Can you work these out from the model? Positions are in its coordinate system, mm. A direction names the side the tool comes from. Coordinates: 2 decimals unless noted, no trailing zeros. Order: outer loops, then holes, each group sorted by start corner. A loop starts at its lowest first (then second) coordinate and runs counter-clockwise, first axis right, second up. Notation, with made-up numbers: (-5, 31) - (42, 31) arc R18 ccw to (42, 62) - close; hole circle Ø4 at (85, -39.5). An arc over 180 degrees is marked (long way). Use a Markdown table: item, result. Add a question column.
(1) I want a section at C-C (y = 3.75). List the corners of the cut face in (x, z) for me, and give its area (3 significant figures).
(2) I want a section at D-D (x = 0). List the corners of the cut face in (y, z) for me, and give its area (3 significant figures).
(3) I want a section at B-B (y = 19). List the corners of the cut face in (x, z) for me.
(4) For pin 1 Ø9 at (x, y) = (-18.5, 7) entering from -Z; pin 2 Ø5 at (y, z) = (18, 35) entering from +X; pin 3 Ø2 at (x, y) = (-27, 7.5) entering from -Z; pin 4 Ø6 at (x, y) = (8.5, 11) entering from +Z, each with a flat end and sliding along its axis, tell me the tip position at first contact or that it passes through.
(5) We'd pull the mould along X, two halves only. Please class faces 5 (the cylindrical face through (25.74, 6.26, 27.16)), 6 (the flat face through (-20.32, 18, 33)), 7 (the flat face through (-15, 22.86, 33)), 8 (the cylindrical face through (1.72, 6.26, -50.77)): pulls with the +X half, pulls with the -X half, needs draft (parallel to the pull), parting line crosses it, or undercut.
(6) If I drill on L1, parallel to X at y = 9.5, z = 0; L2, parallel to Y at x = 42.5, z = 2.5; L3, parallel to X at y = 6.5, z = 6, over which ranges is the centre line in solid material (lowest first)? Write a range as [from, to].
(7) On a 3-axis mill with a long thin cutter (end or side, diameter ignored), from which of +Z, -Z, +X, -X, +Y, -Y can I reach the whole of each face in a straight line? I mean faces 1 (the flat face through (-10.16, 11, 33)), 2 (the flat face through (-15, 0, -36)), 3 (the flat face through (20.32, 18, 33)), 4 (the flat face through (16, 11, 28.137)). Say none if no direction works.
(8) I want a section at A-A (z = 0). List the corners of the cut face in (x, y) for me, and give its area (3 significant figures).
```python
from build123d import *

# Parameters (mm, degrees)
SKETCH1_R           = 50.8
BOSS_EXTRUDE1_DEPTH = 12.7
CUT_EXTRUDE1_DEPTH  = 12.7
SKETCH3_W           = 10.16
SKETCH3_H           = 10.16
BOSS_EXTRUDE2_DEPTH = 10.16
FILLET1_R           = 10.16
FILLET2_R           = 10.16


with BuildPart() as part:
    # Sketch1 → Boss-Extrude1 (new body)
    with BuildSketch(Plane(origin=(0, 0, 0), x_dir=(1, 0, 0), z_dir=(0, 1, 0))):
        Circle(SKETCH1_R)
    extrude(amount=BOSS_EXTRUDE1_DEPTH)

    # Sketch2 → Cut-Extrude1 (cut)
    with BuildSketch(Plane(origin=(0, 12.7, 0), x_dir=(1, 0, 0), z_dir=(0, 1, 0))):
        with BuildLine():
            Line((-25.689206411, -28.136713987), (-10.16, -28.136713987))
            Line((-10.16, -28.136713987), (-10.16, -38.296713987))
            Line((-10.16, -38.296713987), (-33.376663971, -38.296713987))
            ThreePointArc((-33.376663971, -38.296713987), (0, -50.8), (33.376663971, -38.296713987))
            Line((33.376663971, -38.296713987), (10.16, -38.296713987))
            Line((10.16, -38.296713987), (10.16, -28.136713987))
            Line((10.16, -28.136713987), (25.689206411, -28.136713987))
            ThreePointArc((25.689206411, -28.136713987), (0, 38.1), (-25.689206411, -28.136713987))
        make_face()
    extrude(amount=-CUT_EXTRUDE1_DEPTH, mode=Mode.SUBTRACT)

    # Sketch3 → Boss-Extrude2 (add)
    with BuildSketch(Plane(origin=(-12.7, 12.7, 0), x_dir=(0, 0, -1), z_dir=(0, -1, 0))):
        with Locations((-33.216713987, -2.54)):
            Rectangle(SKETCH3_W, SKETCH3_H)
    boss_extrude2 = extrude(amount=-BOSS_EXTRUDE2_DEPTH)

    # Fillet1
    fillet1_edges = [part.edges().sort_by_distance(p)[0] for p in [
        (-25.689206411, 6.35, 28.136713987),
    ]]
    fillet(fillet1_edges, radius=FILLET1_R)

    # Mirror1: Boss-Extrude2 across plane
    add(boss_extrude2.mirror(Plane(origin=(0, 0, 0), x_dir=(0, 0, 1), z_dir=(1, 0, 0))))

    # Fillet2
    fillet2_edges = [part.edges().sort_by_distance(p)[0] for p in [
        (25.689206411, 6.35, 28.136713987),
    ]]
    fillet(fillet2_edges, radius=FILLET2_R)


solid = part.part
```
Answers follow:
| question | item | result |
|---|---|---|
| 1 | outline | (-33.38, 38.3) arc R50.8 ccw (long way) to (33.38, 38.3) - (10.16, 38.3) - (10.16, 28.14) - (21.39, 28.14) arc R10.16 cw to (29.17, 24.51) arc R38.1 cw (long way) to (-29.17, 24.51) arc R10.16 cw to (-21.39, 28.14) - (-10.16, 28.14) - (-10.16, 38.3) - close |
| 1 | area | 3,130 mm² |
| 2 | outline | (0, -50.8) - (12.7, -50.8) - (12.7, -38.1) - (0, -38.1) - close |
| 2 | area | 161 mm² |
| 3 | outline | (-20.32, 28.14) - (-10.16, 28.14) - (-10.16, 38.3) - (-20.32, 38.3) - close; (10.16, 28.14) - (20.32, 28.14) - (20.32, 38.3) - (10.16, 38.3) - close |
| 4 | pin 1 | stops at z = -48.83 |
| 4 | pin 2 | stops at x = 20.32 |
| 4 | pin 3 | stops at z = -43.64 |
| 4 | pin 4 | stops at z = 38.3 |
| 5 | face 5 | undercut |
| 5 | face 6 | pulls with the -X half |
| 5 | face 7 | needs draft |
| 5 | face 8 | parting line crosses it |
| 6 | L1 | x = [-50.8, -38.1], [38.1, 50.8] |
| 6 | L2 | y = [0, 12.7] |
| 6 | L3 | x = [-50.44, -37.62], [37.62, 50.44] |
| 7 | face 1 | +Z, +Y, -Y |
| 7 | face 2 | +Z, -Z, +X, -X, -Y |
| 7 | face 3 | +Z, -Z, +X, +Y |
| 7 | face 4 | +Y, -Y |
| 8 | outline | (-50.8, 0) - (-38.1, 0) - (-38.1, 12.7) - (-50.8, 12.7) - close; (38.1, 0) - (50.8, 0) - (50.8, 12.7) - (38.1, 12.7) - close |
| 8 | area | 323 mm² |
